Source: CAD feature listing. Evaluate the final solid. Frame: model axes, mm. Face numbers are marked on the shaded views. A direction names the side the tool comes from. Coordinates: 2 decimals unless noted, no trailing zeros. Write each loop counter-clockwise with the first axis right and the second up, starting at its lowest first coordinate (ties: lowest second). Pieces come first, ordered by that corner, then holes. Notation, with made-up numbers: M 65,-35 L 103,-35 A17 cw 103,-9 Z; hole C 44,3.25 d6. An arc over 180 degrees is marked long. One line per item, written item: value. Start each with the question number.
Item 1: Cut plane D-D, the plane x = -9. Output: boundary loops of the cut face in (y, z).
Item 2: Cut plane C-C, the plane z = 4.75. Output: boundary loops of the cut face in (x, y), then the cut area to 3 significant figures.
Item 3: Cut plane B-B, the plane z = 0. Output: boundary loops of the cut face in (x, y), then the cut area to 3 significant figures.
Item 4: Set-up query: the marked faces 5 and 6. Return all of +Z, -Z, +X, -X, +Y, -Y with unobstructed straight access to the full face (end or side cutting, diameter ignored); none if empty.
Item 5: Pin query (flat end, axial travel): P1, Ø4, axis at x = -29.5, y = -21.5, coming from the -Z side. Return the tip coordinate at first contact, or that it passes through.
Item 6: Mould query, pull axis X, two halves, no side actions, for the marked faces 1, 2, 3 and 4. Classes: released by +X, released by -X, zero draft, split by the parting line, or undercut.
Item 7: Ray query, L1, parallel to X at y = -10.5, z = 10.5; L2, parallel to Y at x = -42.5, z = 3.75; L3, parallel to X at y = -25, z = 1.5. Return the intervals inside material, ascending. Write a range as from..to.
Item 8: Cut plane A-A, the plane y = -7.25. Output: boundary loops of the cut face in (x, z).
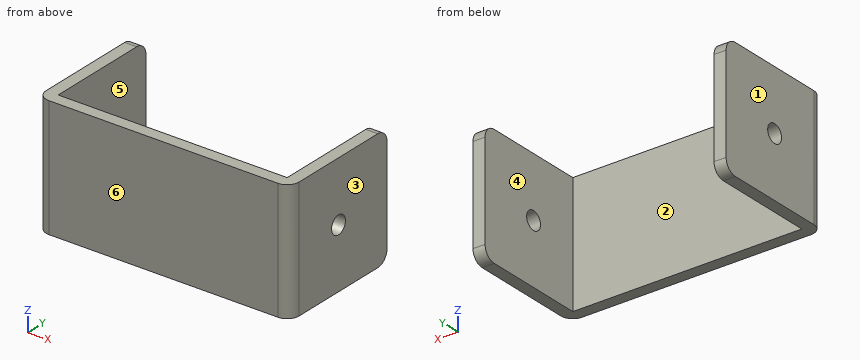
```python
from build123d import *

# Parameters (mm, degrees)
F1_W     = 2.54
F1_H     = 25.4
F3_R     = 1.905
F5_DEPTH = 2.54
F4_R     = 1.905
F6_DEPTH = 2.54
F7_R     = 2.54


with BuildPart() as f2:
    # F2: sweep along a path in F0
    with BuildLine(Plane.XY) as f2_path:
        Line((-50.8, 0), (-50.8, -25.4))
        Line((-50.8, -25.4), (0, -25.4))
        Line((0, -25.4), (0, 0))
    # F1 (on Front) → F2 (sweep)
    with BuildSketch(Plane.XZ):
        Rectangle(F1_W, F1_H)
    sweep(path=f2_path.line, transition=Transition.RIGHT)

    # F3 (on face) → F5 (cut, through all)
    with BuildSketch(Plane.YZ.offset(1.27)):
        with Locations((-13.335, 0)):
            Circle(F3_R)
    extrude(amount=-F5_DEPTH, mode=Mode.SUBTRACT)

    # F4 (on face) → F6 (cut, through all)
    with BuildSketch(Plane(origin=(-52.07, 0, 0), x_dir=(0, -1, 0), z_dir=(-1, 0, 0))):
        with Locations((13.335, 0)):
            Circle(F4_R)
    extrude(amount=-F6_DEPTH, mode=Mode.SUBTRACT)

    # F7
    f7_edges = [f2.edges().sort_by_distance(p)[0] for p in [
        (-50.8, 0, 12.7),
        (-50.8, 0, -12.7),
        (0, 0, -12.7),
        (0, 0, 12.7),
        (1.27, -26.67, 0),
        (-52.07, -26.67, 0),
    ]]
    fillet(f7_edges, radius=F7_R)


solid = f2.part
```
From the geometry:
1. outline: M -26.67,-12.7 L -24.13,-12.7 L -24.13,12.7 L -26.67,12.7 Z
2. outline: M -52.07,-24.13 A2.54 ccw -49.53,-26.67 L -1.27,-26.67 A2.54 ccw 1.27,-24.13 L 1.27,0 L -1.27,0 L -1.27,-24.13 L -49.53,-24.13 L -49.53,0 L -52.07,0 Z
2. area: 255 mm²
3. outline: M -52.07,-24.13 A2.54 ccw -49.53,-26.67 L -1.27,-26.67 A2.54 ccw 1.27,-24.13 L 1.27,-15.24 L -1.27,-15.24 L -1.27,-24.13 L -49.53,-24.13 L -49.53,-15.24 L -52.07,-15.24 Z; M -52.07,-11.43 L -49.53,-11.43 L -49.53,0 L -52.07,0 Z; M -1.27,-11.43 L 1.27,-11.43 L 1.27,0 L -1.27,0 Z
3. area: 236 mm²
4. face 5: +Z, -Z, +Y
4. face 6: +Z, -Z, +X, -X, -Y
5. P1: passes through
6. face 1: released by -X
6. face 2: undercut
6. face 3: released by +X
6. face 4: undercut
7. L1: x = -52.07..-49.53, -1.27..1.27
7. L2: y = -26.67..-24.13
7. L3: x = -51.92..1.12
8. outline: M -52.07,-12.7 L -49.53,-12.7 L -49.53,12.7 L -52.07,12.7 Z; M -1.27,-12.7 L 1.27,-12.7 L 1.27,12.7 L -1.27,12.7 Z
